Answer from the drawing. Dimensions are ordinates in mm from the lowest x, y and z of the part. A direction names the side the tool comes from. Coordinates: 2 decimals unless noted, no trailing zeros. Loops run counter-clockwise (first coordinate to the right, second up) from the corner with the lowest first, then second, coordinate; pieces in that order, holes last. Notation, with made-up numbers: (-21, 75.5) - (-3, 75.5) arc R15 ccw to (-3, 94.5) - close; hole circle Ø2 at (0, 9.25). An arc over 180 degrees is marked (long way). Use one line per item in the form item = value. Start each with the question number.
1) Which of the six approach directions +Z, -Z, +X, -X, +Y, -Y give full straight-line access (tool end or side, diameter ignored) to the marked faces 5, 6 and 7?
2) Each of these flat-tipped pins is pushed along its axis until it touches: P1, Ø3, axis at x = 47.5, z = 44.5, coming from the -Y side; P2, Ø1.5, axis at x = 55, y = 4, coming from the +Z side; P3, Ø1, axis at y = 6.5, z = 16.5, coming from the +X side; P4, Ø1, axis at x = 31.5, y = 1.5, coming from the +Z side (1 decimal). Where does it stop, or does it pass through?
3) A cutting plane is placed at A-A (y = 1.25). Give the vertices of the cut face in (x, z).
4) A cutting plane is placed at B-B (z = 7). Give the vertices of the cut face in (x, y).
5) The mould has two halves that part along Z. Classify the marked faces 1, 2, 3 and 4: released by +Z, released by -Z, zero draft, split by the parting line, or undercut.
6) Consider line 1 (Z direction, x = 62, y = 2.25); line 2 (X direction, y = 4.75, z = 5); line 3 (Z direction, x = 54.5, y = 6.75) (1 decimal). Determine where each line is inside the solid, lowest interval first.
7) A cutting plane is placed at C-C (x = 61). Give the vertices of the cut face in (y, z).
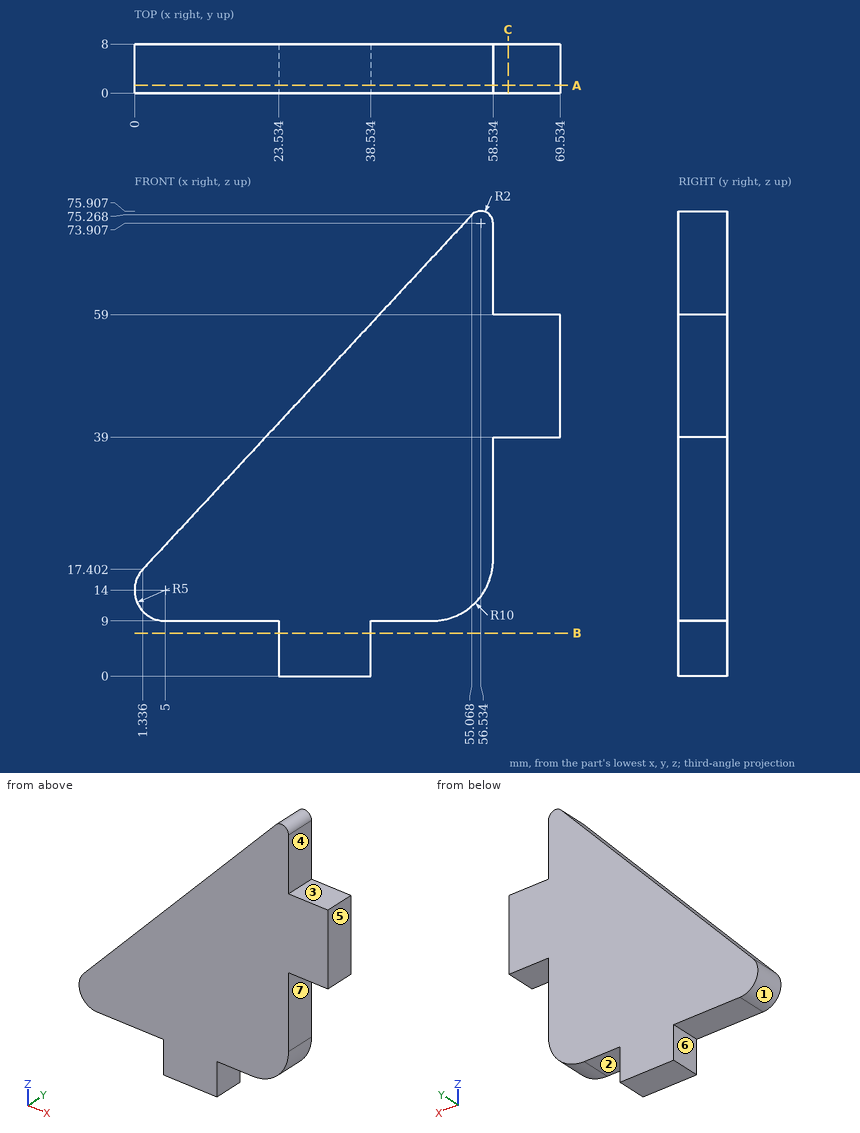
Found:
q1.face_5 = +Z, -Z, +X, +Y, -Y
q1.face_6 = -Z, -X, +Y, -Y
q1.face_7 = -Z, +X, +Y, -Y
q2.P1 = 0
q2.P2 = 75.75
q2.P3 = 58.33
q2.P4 = 50.4
q3.outline = (1.34, 17.4) arc R5 ccw to (5, 9) - (23.53, 9) - (23.53, 0) - (38.53, 0) - (38.53, 9) - (48.53, 9) arc R10 ccw to (58.53, 19) - (58.53, 39) - (69.53, 39) - (69.53, 59) - (58.53, 59) - (58.53, 73.91) arc R2 ccw to (55.07, 75.27) - close
q4.outline = (23.53, 0) - (38.53, 0) - (38.53, 8) - (23.53, 8) - close
q5.face_1 = split by the parting line
q5.face_2 = released by -Z
q5.face_3 = released by +Z
q5.face_4 = zero draft
q6.line_1 = 39 to 59
q6.line_2 = 23.53 to 38.53
q6.line_3 = 11 to 74.7
q7.outline = (0, 39) - (8, 39) - (8, 59) - (0, 59) - close
